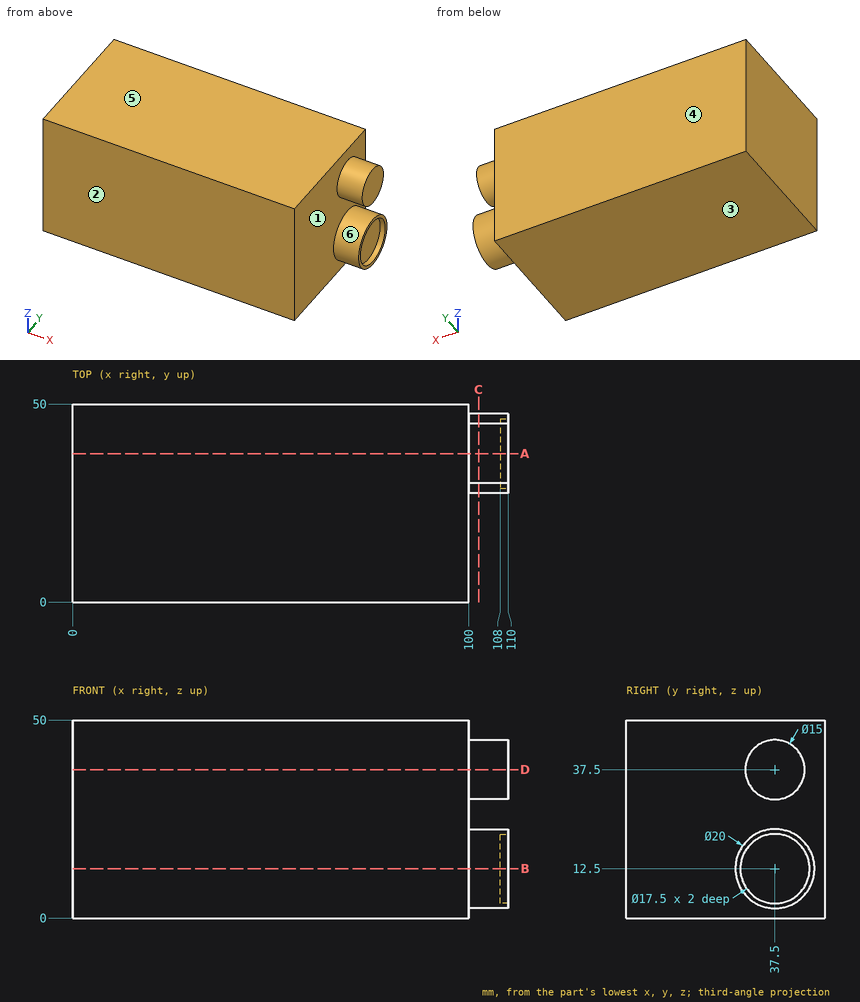
For this review, use the dimensioned drawing (mm, ordinates from the lowest corner) and the shaded views. A direction names the side the tool comes from. Coordinates: 2 decimals unless noted, no trailing zeros. Write each loop counter-clockwise with the first axis right and the second up, starting at its lowest first coordinate (ties: lowest second). Pieces come first, ordered by that corner, then holes. Notation, with made-up numbers: (63.25, 33.25) - (70.25, 33.25) arc R18 cw to (70.25, 66.25) - close; hole circle Ø4 at (44.25, 72.5). An arc over 180 degrees is marked (long way). Answer as a JSON object with one key per item and string values. Group by question number.
1. Mouldability with a two-part tool opening along Z and no side actions: class the marked faces 3, 4, 5 and 6 as pulls with the +Z half, pulls with the -Z half, needs draft (parallel to the pull), parting line crosses it, or undercut.
2. Machinability: for the marked faces 1 and 2, which of the approach directions +Z, -Z, +X, -X, +Y, -Y give a long, thin tool a straight path to every point of the face, cutting with its end or side? Answer none if there is none.
3. Clearance check with a flat-ended pin moving along its axis: pin 1 Ø1.5 at (y, z) = (12, 38) entering from -X. State where the tip first meets the part, or that it passes through.
4. Add section D-D (z = 37.5). Give the boundary of the cut face in (x, y).
5. To check wall thickness, follow probe 1 along Y at (x, z) = (109, 12); probe 2 along X at (y, z) = (18, 44); probe 3 along Y at (x, z) = (100.5, 44). State the ranges of each line that lie inside material, in increasing order.
6. Add section C-C (x = 102.5). Give the boundary of the cut face in (y, z).
7. Add section B-B (z = 12.5). Give the boundary of the cut face in (x, y), plus the area to 4 significant figures.
8. Add section A-A (y = 37.5). Give the boundary of the cut face in (x, z).
Findings:
{
 "1": {"face 3": "pulls with the -Z half", "face 4": "needs draft", "face 5": "pulls with the +Z half", "face 6": "undercut"},
 "2": {"face 1": "+X", "face 2": "+Z, -Z, +X, -X, -Y"},
 "3": {"pin 1": "x = 0"},
 "4": {"outline": "(0, 0) - (100, 0) - (100, 30) - (110, 30) - (110, 45) - (100, 45) - (100, 50) - (0, 50) - close"},
 "5": {"probe 1": "27.51 to 28.76, 46.24 to 47.49", "probe 2": "0 to 100", "probe 3": "33.76 to 41.24"},
 "6": {"outline": "circle Ø20 at (37.5, 12.5); circle Ø15 at (37.5, 37.5)"},
 "7": {"outline": "(0, 0) - (100, 0) - (100, 27.5) - (110, 27.5) - (110, 28.75) - (108, 28.75) - (108, 46.25) - (110, 46.25) - (110, 47.5) - (100, 47.5) - (100, 50) - (0, 50) - close", "area": "5,165 mm²"},
 "8": {"outline": "(0, 0) - (100, 0) - (100, 2.5) - (110, 2.5) - (110, 3.75) - (108, 3.75) - (108, 21.25) - (110, 21.25) - (110, 22.5) - (100, 22.5) - (100, 30) - (110, 30) - (110, 45) - (100, 45) - (100, 50) - (0, 50) - close"}
}
